Work out the finished part from the listing and answer in its coordinate system (mm). Face numbers are marked on the shaded views. A direction names the side the tool comes from. Coordinates: 2 decimals unless noted, no trailing zeros. Loops run counter-clockwise (first coordinate to the right, second up) from the corner with the lowest first, then second, coordinate; pieces in that order, holes last. Notation, with made-up numbers: (-20, -6) - (-9, -6) arc R12 cw to (-9, 12) - close; hole circle Ø5 at (-15, 42). An arc over 180 degrees is marked (long way). Write each question's results on one line, items separated by ' | '. Start each with the question number.
1. A cutting plane is placed at B-B on y = 1. Determine the outline of the cut face in (x, z), then the cut area to 3 significant figures.
2. Which of the six approach directions +Z, -Z, +X, -X, +Y, -Y give full straight-line access (tool end or side, diameter ignored) to the marked faces 1, 2, 3 and 4?
3. A cutting plane is placed at C-C on z = -5. Determine the outline of the cut face in (x, y), then the cut area to 3 significant figures.
4. Each of these flat-tipped pins is pushed along its axis until it touches: P1, Ø5, axis at y = -5.5, z = -10.5, coming from the +X side; P2, Ø4, axis at y = 0.5, z = 25.5, coming from the -X side; P3, Ø6, axis at x = 2.5, z = -10, coming from the -Y side; P4, Ø5, axis at y = 0, z = 26.67, coming from the -X side. Where does it stop, or does it pass through?
5. Determine the mould class of the marked faces 5, 6, 7 and 8 for opening direction Y: released by +Y, released by -Y, zero draft, split by the parting line, or undercut.
6. Find the intervals of material crossed by line 1 along Y through (x, z) = (6.35, 26.67); line 2 along Y through (x, z) = (2.7, 26.67); line 3 along X through (y, z) = (-7, 23.5), in increasing order. Write a range as [from, to].
7. A cutting plane is placed at D-D on z = 25.5. Determine the outline of the cut face in (x, y).
from build123d import *

# Parameters (mm, degrees)
SKETCH2_W                                            = 24.765
SKETCH2_H                                            = 15.875
BOSS_EXTRUDE1_DEPTH                                  = 19.05
SKETCH3_W                                            = 28.575
SKETCH3_H                                            = 22.86
BOSS_EXTRUDE2_DEPTH                                  = 38.1
SKETCH4_W                                            = 14.605
SKETCH4_H                                            = 23.8125
CUT_EXTRUDE1_DEPTH                                   = 47.6725
FILLET5_R                                            = 11.43
FILLET3_R                                            = 6.35
CHAMFER1_SIZE                                        = 5.08
CBORE_FOR_1_4_FILLISTER_HEAD_MACHINE_SCR_D           = 6.4008
CBORE_FOR_1_4_FILLISTER_HEAD_MACHINE_SCR_CBORE_D     = 12.954
CBORE_FOR_1_4_FILLISTER_HEAD_MACHINE_SCR_CBORE_DEPTH = 5.588


with BuildPart() as part:
    # Sketch2 → Boss-Extrude1 (new body)
    with BuildSketch(Plane.XY):
        Rectangle(SKETCH2_W, SKETCH2_H)
    extrude(amount=-BOSS_EXTRUDE1_DEPTH)

    # Sketch3 → Boss-Extrude2 (add)
    with BuildSketch(Plane.XY):
        Rectangle(SKETCH3_W, SKETCH3_H)
    extrude(amount=BOSS_EXTRUDE2_DEPTH)

    # Sketch4 → Cut-Extrude1 (cut, through all)
    with BuildSketch(Plane(origin=(0, -11.43, 0), x_dir=(-1, 0, 0), z_dir=(0, -1, 0))):
        with Locations((6.985, -26.19375)):
            Rectangle(SKETCH4_W, SKETCH4_H)
    extrude(amount=-CUT_EXTRUDE1_DEPTH, mode=Mode.SUBTRACT)

    # Fillet5
    fillet5_edges = [part.edges().sort_by_distance(p)[0] for p in [
        (7.3025, -11.43, 38.1),
        (7.3025, 11.43, 38.1),
    ]]
    fillet(fillet5_edges, radius=FILLET5_R - 0.0001)  # a hair under: the kernel refuses the full size

    # Fillet3
    fillet3_edges = [part.edges().sort_by_distance(p)[0] for p in [
        (-12.3825, 7.9375, -9.525),
        (12.3825, 7.9375, -9.525),
        (12.3825, -7.9375, -9.525),
        (-12.3825, -7.9375, -9.525),
    ]]
    fillet(fillet3_edges, radius=FILLET3_R)

    # Chamfer1
    chamfer1_edges = [part.edges().sort_by_distance(p)[0] for p in [
        (-6.985, 11.43, 14.2875),
        (-6.985, -11.43, 14.2875),
    ]]
    chamfer(chamfer1_edges, length=CHAMFER1_SIZE)

    # CBORE for 1/4 Fillister Head Machine Screw1 (through all)
    with Locations(Plane(origin=(14.2875, 0, 26.67), x_dir=(0, 0, 1), z_dir=(1, 0, 0))):
        with Locations((0, 0)):
            cbore_for_1_4_fillister_head_machine_scr = CounterBoreHole(CBORE_FOR_1_4_FILLISTER_HEAD_MACHINE_SCR_D / 2, CBORE_FOR_1_4_FILLISTER_HEAD_MACHINE_SCR_CBORE_D / 2, CBORE_FOR_1_4_FILLISTER_HEAD_MACHINE_SCR_CBORE_DEPTH)

    # Mirror1: CBORE for 1/4 Fillister Head Machine Screw1 across plane
    add(cbore_for_1_4_fillister_head_machine_scr.mirror(Plane(origin=(6.985, 0, 0), x_dir=(0, 0, 1), z_dir=(1, 0, 0))), mode=Mode.SUBTRACT)


solid = part.part
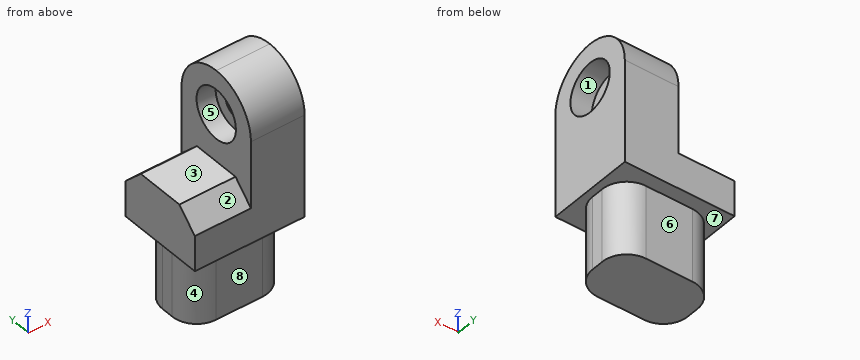
Values:
1) outline: (-14.29, 0) - (-12.38, 0) - (-12.38, -19.05) - (12.38, -19.05) - (12.38, 0) - (14.29, 0) - (14.29, 20.27) - (8.7, 20.27) - (8.7, 23.63) - (5.27, 23.63) - (5.27, 20.27) - (0.32, 20.27) - (0.32, 14.29) - (-14.29, 14.29) - close; (0.32, 33.07) - (5.27, 33.07) - (5.27, 29.71) - (8.7, 29.71) - (8.7, 33.07) - (14.29, 33.07) - (14.29, 38.06) - (0.32, 38.06) - close | area: 1,060 mm^2
2) face 1: +X | face 2: +Z, -X, -Y | face 3: +Z, -X, +Y, -Y | face 4: -Z, -X, -Y
3) outline: (-12.38, -1.59) arc R6.35 ccw to (-6.03, -7.94) - (6.03, -7.94) arc R6.35 ccw to (12.38, -1.59) - (12.38, 1.59) arc R6.35 ccw to (6.03, 7.94) - (-6.03, 7.94) arc R6.35 ccw to (-12.38, 1.59) - close | area: 359 mm^2
4) P1: x = 12.22 | P2: x = 5.27 | P3: y = -7.94 | P4: through
5) face 5: undercut | face 6: released by +Y | face 7: zero draft | face 8: released by -Y
6) line 1: [-11.43, -3.2], [3.2, 11.43] | line 2: [-11.43, -6.48], [6.48, 11.43] | line 3: [0.32, 14.29]
7) outline: (0.32, -11.43) - (14.29, -11.43) - (14.29, -6.37) - (8.7, -6.37) - (8.7, -2.98) - (5.27, -2.98) - (5.27, -6.37) - (0.32, -6.37) - close; (0.32, 6.37) - (5.27, 6.37) - (5.27, 2.98) - (8.7, 2.98) - (8.7, 6.37) - (14.29, 6.37) - (14.29, 11.43) - (0.32, 11.43) - close
